Input: part model. Units: mm. Frame: model coordinates. A direction names the side the tool comes from. Round coordinates to 2 decimals unless told otherwise and drop trailing zeros. Order: outer loops, then holes, each group sorted by start corner. A loop starts at its lowest first (then second) coordinate and runs counter-clockwise, first axis right, second up. Notation, with made-up numbers: M 76.5,19 L 111.5,19 A21 cw 111.5,30 Z; hole C -35,34.5 d10. An arc over 180 degrees is marked long. One line per question, with ' | ' between items.
```python
from build123d import *

# Parameters (mm, degrees)
F1_DEPTH = 7.0358


with BuildPart() as f1:
    # F0 (on Top) → F1 (new body)
    with BuildSketch(Plane.XY):
        with BuildLine():
            Line((-9.5577161638, 50.7395111935), (-9.5577161638, 17.7112849253))
            Line((-9.5577161638, 17.7112849253), (0, 46.55185))
            Line((0, 46.55185), (0, 51.63185))
            ThreePointArc((0, 51.63185), (-4.799640789, 51.408281266), (-9.5577161638, 50.7395111935))
        make_face()
        with BuildLine():
            Line((0, 46.55185), (9.5577161638, 17.7112849253))
            Line((9.5577161638, 17.7112849253), (9.5577161638, 50.7395111935))
            ThreePointArc((9.5577161638, 50.7395111935), (4.799640789, 51.408281266), (0, 51.63185))
            Line((0, 51.63185), (0, 46.55185))
        make_face()
        with BuildLine():
            Line((9.5577161638, 17.7112849253), (9.5577161638, 10.636620877))
            ThreePointArc((9.5577161638, 10.636620877), (12.3840918707, 7.1499587752), (13.9904419718, 2.9589145615))
            Line((13.9904419718, 2.9589145615), (20.1172807609, -0.5784174627))
            ThreePointArc((20.1172807609, -0.5784174627), (20.1235159205, -0.2892386033), (20.1255944502, 0))
            ThreePointArc((20.1255944502, 0), (17.282856699, 10.3122459385), (9.5577161638, 17.7112849253))
        make_face()
        with BuildLine():
            Line((10.5595645971, -17.1328674627), (4.432725808, -13.5955354385))
            ThreePointArc((4.432725808, -13.5955354385), (0, -14.2999175504), (-4.432725808, -13.5955354385))
            Line((-4.432725808, -13.5955354385), (-10.5595645971, -17.1328674627))
            ThreePointArc((-10.5595645971, -17.1328674627), (0, -20.1255944502), (10.5595645971, -17.1328674627))
        make_face()
        with BuildLine():
            Line((-20.1172807609, -0.5784174627), (-13.9904419718, 2.9589145615))
            ThreePointArc((-13.9904419718, 2.9589145615), (-12.3840918707, 7.1499587752), (-9.5577161638, 10.636620877))
            Line((-9.5577161638, 10.636620877), (-9.5577161638, 17.7112849253))
            ThreePointArc((-9.5577161638, 17.7112849253), (-17.4292760601, 10.0627972251), (-20.1172807609, -0.5784174627))
        make_face()
        with BuildLine():
            Line((-48.7205637511, -17.0925305967), (-20.1172807609, -0.5784174627))
            ThreePointArc((-20.1172807609, -0.5784174627), (-17.4292760601, 10.0627972251), (-9.5577161638, 17.7112849253))
            Line((-9.5577161638, 17.7112849253), (-9.5577161638, 50.7395111935))
            ThreePointArc((-9.5577161638, 50.7395111935), (-9.5602138637, 50.7390406423), (-9.5627115404, 50.7385699682))
            ThreePointArc((-9.5627115404, 50.7385699682), (-20.2584374888, 11.6962143375), (-48.7222463144, -17.087733861))
            ThreePointArc((-48.7222463144, -17.087733861), (-48.7214050917, -17.0901322496), (-48.7205637511, -17.0925305967))
        make_face()
        with BuildLine():
            Line((9.5577161638, 50.7395111935), (9.5577161638, 17.7112849253))
            ThreePointArc((9.5577161638, 17.7112849253), (17.282856699, 10.3122459385), (20.1255944502, 0))
            ThreePointArc((20.1255944502, 0), (20.1235159205, -0.2892386033), (20.1172807609, -0.5784174627))
            Line((20.1172807609, -0.5784174627), (45.0939427751, -14.9987))
            Line((45.0939427751, -14.9987), (48.7205637511, -17.0925305967))
            ThreePointArc((48.7205637511, -17.0925305967), (48.7214050917, -17.0901322496), (48.7222463144, -17.087733861))
            ThreePointArc((48.7222463144, -17.087733861), (20.2584374888, 11.6962143375), (9.5627115404, 50.7385699682))
            ThreePointArc((9.5627115404, 50.7385699682), (9.5602138637, 50.7390406423), (9.5577161638, 50.7395111935))
        make_face()
        with BuildLine():
            Line((35.5362266113, -31.55315), (10.5595645971, -17.1328674627))
            ThreePointArc((10.5595645971, -17.1328674627), (0, -20.1255944502), (-10.5595645971, -17.1328674627))
            Line((-10.5595645971, -17.1328674627), (-39.1628475873, -33.6469805967))
            ThreePointArc((-39.1628475873, -33.6469805967), (-39.1611912281, -33.6489083927), (-39.1595347739, -33.6508361072))
            ThreePointArc((-39.1595347739, -33.6508361072), (0, -23.392428675), (39.1595347739, -33.6508361072))
            ThreePointArc((39.1595347739, -33.6508361072), (39.1611912281, -33.6489083927), (39.1628475873, -33.6469805967))
            Line((39.1628475873, -33.6469805967), (35.5362266113, -31.55315))
        make_face()
        with BuildLine():
            Line((-39.1628475873, -33.6469805967), (-10.5595645971, -17.1328674627))
            Line((-10.5595645971, -17.1328674627), (-40.3150846932, -23.275925))
            Line((-40.3150846932, -23.275925), (-44.7144937444, -25.815925))
            ThreePointArc((-44.7144937444, -25.815925), (-42.1210571467, -29.8607514853), (-39.1628475873, -33.6469805967))
        make_face()
        with BuildLine():
            Line((-40.3150846932, -23.275925), (-20.1172807609, -0.5784174627))
            Line((-20.1172807609, -0.5784174627), (-48.7205637511, -17.0925305967))
            ThreePointArc((-48.7205637511, -17.0925305967), (-46.9206979357, -21.5475297807), (-44.7144937444, -25.815925))
            Line((-44.7144937444, -25.815925), (-40.3150846932, -23.275925))
        make_face()
        Polygon((40.3150846932, -23.275925), (10.5595645971, -17.1328674627), (35.5362266113, -31.55315), (37.7359311369, -27.74315), align=None)
        Polygon((45.0939427751, -14.9987), (20.1172807609, -0.5784174627), (40.3150846932, -23.275925), (42.5539427751, -19.3981090512), align=None)
        with BuildLine():
            Line((-4.432725808, -13.5955354385), (0, -11.0363))
            ThreePointArc((0, -11.0363), (-5.51815, -9.5577161638), (-9.5577161638, -5.51815))
            ThreePointArc((-9.5577161638, -5.51815), (-11.0363, 0), (-9.5577161638, 5.51815))
            Line((-9.5577161638, 5.51815), (-13.9904419718, 2.9589145615))
            ThreePointArc((-13.9904419718, 2.9589145615), (-12.3840918707, -7.1499587752), (-4.432725808, -13.5955354385))
        make_face()
        with BuildLine():
            Line((-13.9904419718, 2.9589145615), (-9.5577161638, 5.51815))
            Line((-9.5577161638, 5.51815), (-9.5577161638, 10.636620877))
            ThreePointArc((-9.5577161638, 10.636620877), (-12.3840918707, 7.1499587752), (-13.9904419718, 2.9589145615))
        make_face()
        with BuildLine():
            ThreePointArc((0, 11.0363), (5.51815, 9.5577161638), (9.5577161638, 5.51815))
            Line((9.5577161638, 5.51815), (9.5577161638, 10.636620877))
            ThreePointArc((9.5577161638, 10.636620877), (0, 14.2999175504), (-9.5577161638, 10.636620877))
            Line((-9.5577161638, 10.636620877), (-9.5577161638, 5.51815))
            ThreePointArc((-9.5577161638, 5.51815), (-5.51815, 9.5577161638), (0, 11.0363))
        make_face()
        with BuildLine():
            Line((9.5577161638, 10.636620877), (9.5577161638, 5.51815))
            Line((9.5577161638, 5.51815), (13.9904419718, 2.9589145615))
            ThreePointArc((13.9904419718, 2.9589145615), (12.3840918707, 7.1499587752), (9.5577161638, 10.636620877))
        make_face()
        with BuildLine():
            ThreePointArc((11.0363, 0), (10.6602471967, -2.8564046275), (9.5577161638, -5.51815))
            ThreePointArc((9.5577161638, -5.51815), (5.51815, -9.5577161638), (0, -11.0363))
            Line((0, -11.0363), (4.432725808, -13.5955354385))
            ThreePointArc((4.432725808, -13.5955354385), (11.5731425189, -8.3994055852), (14.2999175504, 0))
            ThreePointArc((14.2999175504, 0), (14.2223382156, 1.487527354), (13.9904419718, 2.9589145615))
            Line((13.9904419718, 2.9589145615), (9.5577161638, 5.51815))
            ThreePointArc((9.5577161638, 5.51815), (10.6602471967, 2.8564046275), (11.0363, 0))
        make_face()
        with BuildLine():
            Line((4.432725808, -13.5955354385), (0, -11.0363))
            Line((0, -11.0363), (-4.432725808, -13.5955354385))
            ThreePointArc((-4.432725808, -13.5955354385), (0, -14.2999175504), (4.432725808, -13.5955354385))
        make_face()
        with BuildLine():
            Line((37.7359311369, -27.74315), (35.5362266113, -31.55315))
            Line((35.5362266113, -31.55315), (39.1628475873, -33.6469805967))
            ThreePointArc((39.1628475873, -33.6469805967), (42.1210570839, -29.8607515739), (44.7144936357, -25.8159251882))
            ThreePointArc((44.7144936357, -25.8159251882), (46.9206978904, -21.5475298794), (48.7205637511, -17.0925305967))
            Line((48.7205637511, -17.0925305967), (45.0939427751, -14.9987))
            Line((45.0939427751, -14.9987), (42.5539427751, -19.3981090512))
            Line((42.5539427751, -19.3981090512), (40.3150846932, -23.275925))
            Line((40.3150846932, -23.275925), (37.7359311369, -27.74315))
        make_face()
    extrude(amount=F1_DEPTH)


solid = f1.part
```
Item 1: Access query for faces 4 (the flat face through (-4.846, 31.93, 3.469)), 5 (the flat face through (11, -3, 0)). Directions: +Z, -Z, +X, -X, +Y, -Y. A direction counts if a zero-diameter tool reaches every point of the face in a straight line with its end or side. Return the directions, or none.
Report:
face 4: +Z, -Z | face 5: -Z, +X, -X, +Y, -Y
Item 2: First-contact query: pin 1 (2 mm diameter, centred on x = -14, z = 2, fed in from -Y); pin 2 (2 mm diameter, centred on y = 14, z = 3, fed in from -X); pin 3 (2 mm diameter, centred on y = -22.5, z = 5, fed in from +X). Flat tips, straight axial feed; report the tip coordinate or a pass-through.
Report:
pin 1: y = -24.81 | pin 2: x = -19.52 | pin 3: x = 46.94
Item 3: Section query C-C, the plane y = -9. Return loops of the section in (x, z).
Report:
outline: M -37.44,0 L -27.61,0 L -27.61,7.04 L -37.44,7.04 Z; M -11.11,0 L -6.39,0 L -6.39,7.04 L -11.11,7.04 Z; M 6.39,0 L 11.11,0 L 11.11,7.04 L 6.39,7.04 Z; M 27.61,0 L 37.44,0 L 37.44,7.04 L 27.61,7.04 Z
Item 4: Section query D-D, the plane x = -16. Return loops of the section in (y, z), plus the area to 3 significant figures.
Report:
outline: M -25.01,0 L -18.26,0 L -18.26,7.04 L -25.01,7.04 Z; M 1.8,0 L 20.21,0 L 20.21,7.04 L 1.8,7.04 Z | area: 177 mm²
Item 5: Line query: line 1 along X through (y, z) = (15, 2.25); line 2 along Y through (x, z) = (-40, 4); line 3 along X through (y, z) = (42, 4.75). Output: solid intervals per line, ascending. Write a range as from..to.
Report:
line 1: -18.45..-9.56, 9.56..18.45 | line 2: -32.65..-23.21, -22.92..-11.11 | line 3: -10.14..-1.51, 1.51..10.14
Item 6: Section query B-B, the plane x = -5.5. Return loops of the section in (y, z), plus the area to 3 significant figures.
Report:
outline: M -23.58,0 L -14.21,0 L -14.21,7.04 L -23.58,7.04 Z; M -13.2,0 L -9.57,0 L -9.57,7.04 L -13.2,7.04 Z; M 9.57,0 L 13.2,0 L 13.2,7.04 L 9.57,7.04 Z; M 29.96,0 L 51.34,0 L 51.34,7.04 L 29.96,7.04 Z | area: 267 mm²
Item 7: Section query A-A, the plane y = 22.5. Return loops of the section in (x, z), plus the area to 3 significant figures.
Report:
outline: M -15.06,0 L -7.97,0 L -7.97,7.04 L -15.06,7.04 Z; M 7.97,0 L 15.06,0 L 15.06,7.04 L 7.97,7.04 Z | area: 99.8 mm²
Item 8: Mould query, pull axis X, two halves, no side actions, for faces 1 (the cylindrical face through (20.547, 11.201, 3.469)), 2 (the flat face through (-7.453, -15.339, 3.469)), 3 (the cylindrical face through (-19.974, 12.193, 3.469)). Classes: +X half, -X half, draft (parallel to the pull), parting line (faces both ways), or undercut.
Report:
face 1: +X half | face 2: undercut | face 3: -X half
